Input: part model. Units: mm. Frame: model coordinates. Face numbers are marked on the shaded views. A direction names the side the tool comes from. Give positions to 0.01 mm unless a question says otherwise; leave off trailing zeros. Order: outer loops, then holes, each group sorted by start corner. A loop starts at its lowest first (then second) coordinate and runs counter-clockwise, first axis right, second up. Notation, with made-up numbers: (61.5, 80.25) -> (66.5, 80.25) arc R29 ccw to (66.5, 108.25) -> close; hole circle Ø4 at (44.5, 88.5). An arc over 180 degrees is marked (long way). Use a Markdown table: item, result. Add a question column.
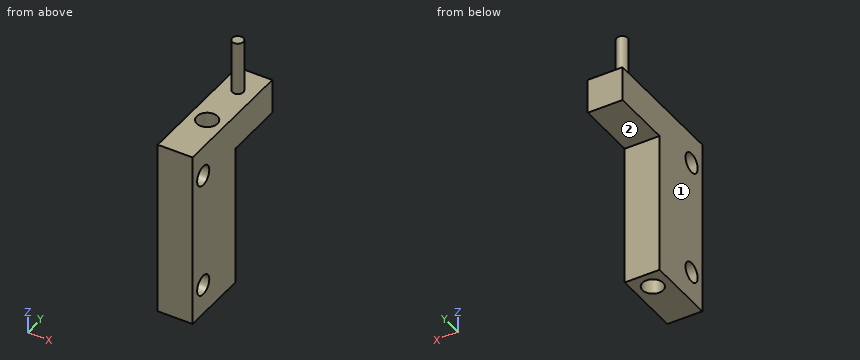
from build123d import *

# Parameters (mm, degrees)
SKETCH2_W           = 15
SKETCH2_H           = 30
SKETCH2_R           = 4.45
BOSS_EXTRUDE1_DEPTH = 76.2
SKETCH3_R           = 4.25
CUT_EXTRUDE2_DEPTH  = 16
SKETCH5_W           = 15
SKETCH5_H           = 26
BOSS_EXTRUDE3_DEPTH = 15
SKETCH8_R           = 2.4
BOSS_EXTRUDE4_DEPTH = 23


with BuildPart() as part:
    # Sketch2 → Boss-Extrude1 (new body)
    with BuildSketch(Plane.XY):
        with Locations((-10.953990987, 24.19276181)):
            Rectangle(SKETCH2_W, SKETCH2_H)
        with Locations((-10.953990987, 31.69276181)):
            Circle(SKETCH2_R, mode=Mode.SUBTRACT)
    extrude(amount=BOSS_EXTRUDE1_DEPTH)

    # Sketch3 → Cut-Extrude2 (cut, through all)
    with BuildSketch(Plane(origin=(-3.453990987, 0, 0), x_dir=(0, 0, -1), z_dir=(1, 0, 0))):
        with Locations((-63.1, 16.69276181)):
            Circle(SKETCH3_R)
        with Locations((-13.1, 16.69276181)):
            Circle(SKETCH3_R)
    extrude(amount=-CUT_EXTRUDE2_DEPTH, mode=Mode.SUBTRACT)

    # Sketch5 → Boss-Extrude3 (add)
    with BuildSketch(Plane.XY.offset(76.2)):
        with Locations((-10.953990987, 52.19276181)):
            Rectangle(SKETCH5_W, SKETCH5_H)
    extrude(amount=-BOSS_EXTRUDE3_DEPTH)

    # Sketch8 → Boss-Extrude4 (add)
    with BuildSketch(Plane.XY.offset(76.2)):
        with Locations((-10.953990987, 53.19276181)):
            Circle(SKETCH8_R)
    extrude(amount=BOSS_EXTRUDE4_DEPTH)


solid = part.part
Q1. Section query D-D (z = 63). Return loops of the section in (x, y), plus the area to 3 significant figures.
Q2. Section query B-B (x = -7.5). Return loops of the section in (y, z), plus the area to 3 significant figures.
Q3. Ray query, line 1 (Y direction, x = -8.5, z = 13.1); line 2 (Y direction, x = -13.75, z = 13.1); line 3 (Z direction, x = -16, y = 53.5). Return the intervals inside material, ascending.
Q4. Section query C-C (y = 18). Return loops of the section in (x, z).
Q5. Section query A-A (z = 13.1). Return loops of the section in (x, y), plus the area to 3 significant figures.
Q6. First-contact query: pin 1 (6 mm diameter, centred on x = -7, y = 48.5, fed in from +Z); pin 2 (7 mm diameter, centred on y = 16.69, z = 63.1, fed in from +X); pin 3 (6 mm diameter, centred on y = 55, z = 88, fed in from +X). Flat tips, straight axial feed; report the tip coordinate or a pass-through.
Q7. Access query for the marked faces 1 and 2. Directions: +Z, -Z, +X, -X, +Y, -Y. A direction counts if a zero-diameter tool reaches every point of the face in a straight line with its end or side. Return the directions, or none.
Solution:
| question | item | result |
|---|---|---|
| 1 | outline | (-18.45, 9.19) -> (-3.45, 9.19) -> (-3.45, 12.44) -> (-18.45, 12.44) -> close; (-18.45, 20.94) -> (-3.45, 20.94) -> (-3.45, 65.19) -> (-18.45, 65.19) -> close; hole circle Ø8.9 at (-10.95, 31.69) |
| 1 | area | 650 mm² |
| 2 | outline | (9.19, 0) -> (28.89, 0) -> (28.89, 76.2) -> (9.19, 76.2) -> close; (34.5, 0) -> (39.19, 0) -> (39.19, 61.2) -> (65.19, 61.2) -> (65.19, 76.2) -> (34.5, 76.2) -> close; hole circle Ø8.5 at (16.69, 13.1); hole circle Ø8.5 at (16.69, 63.1) |
| 2 | area | 2,130 mm² |
| 3 | line 1 | y = 9.19 to 12.44, 20.94 to 27.98, 35.4 to 39.19 |
| 3 | line 2 | y = 9.19 to 12.44, 20.94 to 28.23, 35.15 to 39.19 |
| 3 | line 3 | z = 61.2 to 76.2 |
| 4 | outline | (-18.45, 0) -> (-3.45, 0) -> (-3.45, 9.06) -> (-18.45, 9.06) -> close; (-18.45, 17.14) -> (-3.45, 17.14) -> (-3.45, 59.06) -> (-18.45, 59.06) -> close; (-18.45, 67.14) -> (-3.45, 67.14) -> (-3.45, 76.2) -> (-18.45, 76.2) -> close |
| 5 | outline | (-18.45, 9.19) -> (-3.45, 9.19) -> (-3.45, 12.44) -> (-18.45, 12.44) -> close; (-18.45, 20.94) -> (-3.45, 20.94) -> (-3.45, 39.19) -> (-18.45, 39.19) -> close; hole circle Ø8.9 at (-10.95, 31.69) |
| 5 | area | 260 mm² |
| 6 | pin 1 | stops at z = 76.2 |
| 6 | pin 2 | passes through |
| 6 | pin 3 | stops at x = -8.55 |
| 7 | face 1 | +Z, -Z, -X, +Y, -Y |
| 7 | face 2 | -Z, +X, -X, +Y |
